```python
from build123d import *

# Parameters (mm, degrees)
SKETCH26_R                       = 27.463437659
BOSS_EXTRUDE1_DEPTH              = 5
SKETCH27_R                       = 25.998508152
CUT_EXTRUDE1_DEPTH               = 5
F_0_55_0_55_DIAMETER_HOLE2_D     = 1.17
F_0_55_0_55_DIAMETER_HOLE2_DEPTH = 2
F_0_55_0_55_DIAMETER_HOLE2_TIP   = 0.351503462
F_0_55_0_55_DIAMETER_HOLE4_D     = 1.17
F_0_55_0_55_DIAMETER_HOLE4_DEPTH = 2
F_0_55_0_55_DIAMETER_HOLE4_TIP   = 0.351503462


with BuildPart() as part:
    # Sketch23 → Revolve3 (revolve)
    with BuildSketch(Plane(origin=(0, 0, 0), x_dir=(-1, 0, 0), z_dir=(0, 0, -1)), mode=Mode.PRIVATE) as revolve3_sk:
        Polygon((0, 24.895699348), (-27.463437659, 24.895699348), (-14.091987401, 5.799289315), (0, 5.799289315), align=None)
    revolve(revolve3_sk.sketch.rotate(Axis((0, 0, 0), (0, 1, 0)), 90), axis=Axis((0, 0, 0), (0, 1, 0)))

    # Sketch25 → Cut-Revolve3 (revolve, cut)
    with BuildSketch(Plane(origin=(0, 0, 0), x_dir=(-1, 0, 0), z_dir=(0, 0, -1)), mode=Mode.PRIVATE) as cut_revolve3_sk:
        Polygon((0, 30), (-29.6127402, 30.057357644), (-10.448606131, 2.688137772), (0, 2.666892546), align=None)
    revolve(cut_revolve3_sk.sketch.rotate(Axis((0, 0, 0), (0, 1, 0)), 270), axis=Axis((0, 0, 0), (0, 1, 0)), mode=Mode.SUBTRACT)

    # Sketch26 → Boss-Extrude1 (add)
    with BuildSketch(Plane(origin=(0, 24.895699348, 0), x_dir=(1, 0, 0), z_dir=(0, 1, 0))):
        with Locations(Location((0, 0, 0), (0, 0, 270))):
            Circle(SKETCH26_R)
    extrude(amount=BOSS_EXTRUDE1_DEPTH)

    # Sketch27 → Cut-Extrude1 (cut)
    with BuildSketch(Plane(origin=(0, 29.895699348, 0), x_dir=(1, 0, 0), z_dir=(0, 1, 0))):
        with Locations(Location((0, 0, 0), (0, 0, 270))):
            Circle(SKETCH27_R)
    extrude(amount=-CUT_EXTRUDE1_DEPTH, mode=Mode.SUBTRACT)

    # Ø0.55 (0.55) Diameter Hole2
    with Locations(Plane(origin=(17.902646224, 14.36906592, 9.121853864), x_dir=(0.617893015445, 0.786262183666, 0), z_dir=(0.729869815764, -0.573576436351, 0.371887245949))):
        with Locations((0, 0)):
            Hole(F_0_55_0_55_DIAMETER_HOLE2_D / 2, depth=F_0_55_0_55_DIAMETER_HOLE2_DEPTH)
            with Locations((0, 0, -(F_0_55_0_55_DIAMETER_HOLE2_DEPTH + F_0_55_0_55_DIAMETER_HOLE2_TIP / 2))):  # 118° drill point
                Cone(0, F_0_55_0_55_DIAMETER_HOLE2_D / 2, F_0_55_0_55_DIAMETER_HOLE2_TIP, mode=Mode.SUBTRACT)

    # Ø0.55 (0.55) Diameter Hole4
    with Locations(Plane(origin=(-17.902646224, 14.36906592, -9.121853864), x_dir=(0.617893015445, -0.786262183666, 0), z_dir=(-0.729869815764, -0.573576436351, -0.371887245949))):
        with Locations((0, 0)):
            Hole(F_0_55_0_55_DIAMETER_HOLE4_D / 2, depth=F_0_55_0_55_DIAMETER_HOLE4_DEPTH)
            with Locations((0, 0, -(F_0_55_0_55_DIAMETER_HOLE4_DEPTH + F_0_55_0_55_DIAMETER_HOLE4_TIP / 2))):  # 118° drill point
                Cone(0, F_0_55_0_55_DIAMETER_HOLE4_D / 2, F_0_55_0_55_DIAMETER_HOLE4_TIP, mode=Mode.SUBTRACT)


solid = part.part
```
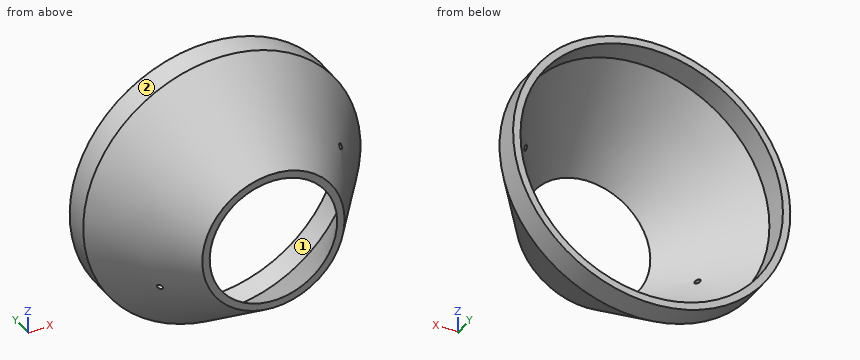
Input: part model. Units: mm. Frame: model coordinates. Face numbers are marked on the shaded views. Give positions to 0.01 mm unless a question says otherwise; leave off trailing zeros. Order: outer loops, then holes, each group sorted by start corner. A loop starts at its lowest first (then second) coordinate and runs counter-clockwise, first axis right, second up.
1. Mould query, pull axis X, two halves, no side actions, for the marked faces 1 and 2. Classes: released by +X, released by -X, zero draft, split by the parting line, or undercut.
Derived:
face 1: undercut
face 2: split by the parting line
2. Material intervals for L1, parallel to X at y = 26.7, z = 0; L2, parallel to Z at x = -9.5, y = 13; L3, parallel to X at y = 16.25, z = -9.5, sorted ascending.
Derived:
L1: x = -27.46 to -26, 26 to 27.46
L2: z = -16.61 to -14.9, 14.9 to 16.61
L3: x = -19.19 to -17.54, 17.54 to 19.19
3. Section C-C on y = 11.5. Return the cut outline in (x, z), and give its area (3 significant figures).
Derived:
outline: circle Ø36.17 at (0, 0); hole circle Ø33.24 at (0, 0)
area: 160 mm2
4. Section B-B on x = 0. Return the cut outline in (y, z).
Derived:
outline: (5.8, -14.09) - (24.9, -27.46) - (29.9, -27.46) - (29.9, -26) - (24.9, -26) - (5.8, -12.63) - close; (5.8, 12.63) - (24.9, 26) - (29.9, 26) - (29.9, 27.46) - (24.9, 27.46) - (5.8, 14.09) - close
5. Pin query (flat end, axial travel): pin 1 (1 mm diameter, centred on x = -3.5, y = 18.5, fed in from +Z); pin 2 (6 mm diameter, centred on y = 23, z = -3, fed in from +X); pin 3 (5 mm diameter, centred on y = 12, z = 16, fed in from +X). Return the tip coordinate at first contact, or that it passes through.
Derived:
pin 1: stops at z = 23.08
pin 2: stops at x = 27.46
pin 3: stops at x = 13.58
6. Section D-D on y = 7.5. Return the cut outline in (x, z), and give its area (3 significant figures).
Derived:
outline: circle Ø30.57 at (0, 0); hole circle Ø27.64 at (0, 0)
area: 134 mm2
7. Section A-A on z = 0. Return the cut outline in (x, y).
Derived:
outline: (-27.46, 24.9) - (-14.09, 5.8) - (-12.63, 5.8) - (-26, 24.9) - (-26, 29.9) - (-27.46, 29.9) - close; (12.63, 5.8) - (14.09, 5.8) - (27.46, 24.9) - (27.46, 29.9) - (26, 29.9) - (26, 24.9) - close
